Part model, mm, in its own coordinate system. A direction names the side the tool comes from. Give positions to 0.01 mm unless a question says otherwise; leave off trailing zeros. Loops run counter-clockwise (first coordinate to the right, second up) from the corner with the lowest first, then second, coordinate; pieces in that order, holes last. Notation, with made-up numbers: M -15.75,50.25 L 35.25,50.25 A17 ccw 35.25,72.25 Z; hole C 62,-5.5 d10. An arc over 180 degrees is marked long. Answer in a Markdown table with one row per item.
from build123d import *

# Parameters (mm, degrees)
SKETCH_W     = 12.8
SKETCH_H     = 9.8
PAD_DEPTH    = 10
SKETCH001_W  = 15
SKETCH001_H  = 12
PAD001_DEPTH = 1
CHAMFER_SIZE = 1


with BuildPart() as part:
    # Sketch → Pad (new body)
    with BuildSketch(Plane.XZ):
        Rectangle(SKETCH_W, SKETCH_H)
    extrude(amount=PAD_DEPTH)

    # Sketch001 (on Face1 of Pad) → Pad001 (join)
    with BuildSketch(Plane(origin=(0, 0, 4.9), x_dir=(-1, 0, 0), z_dir=(0, 0, 1))):
        with Locations((-0.066966, 5)):
            Rectangle(SKETCH001_W, SKETCH001_H)
    extrude(amount=PAD001_DEPTH)

    # Chamfer
    chamfer_edges = [part.edges().sort_by_distance(p)[0] for p in [
        (-6.4, -10, 0),
        (0, -10, -4.9),
        (-6.4, -5, -4.9),
        (-6.4, 0, 0),
        (6.4, -10, 0),
        (6.4, -5, -4.9),
        (6.4, 0, 0),
        (0, 0, -4.9),
    ]]
    chamfer(chamfer_edges, length=CHAMFER_SIZE)


solid = part.part
(1) Pin check, flat tips, straight feed: pin 1 Ø4.5 at (x, z) = (2.5, 0.5) entering from -Y; pin 2 Ø2.5 at (y, z) = (-6, 2.5) entering from -X; pin 3 Ø2 at (x, z) = (0.5, 3.5) entering from +Y. Stop position of each tip, or through.
Recorded:
| item | result |
|---|---|
| pin 1 | stops at y = -10 |
| pin 2 | stops at x = -6.4 |
| pin 3 | stops at y = 0 |
(2) Saw through at C-C (x = -1.5). Write the cut outline in (y, z).
Recorded:
| item | result |
|---|---|
| outline | M -11,4.9 L -10,4.9 L -10,-3.9 L -9,-4.9 L -1,-4.9 L 0,-3.9 L 0,4.9 L 1,4.9 L 1,5.9 L -11,5.9 Z |
(3) Drill centre lines: line 1 along Y through (x, z) = (2.25, 4.5); line 2 along X through (y, z) = (-8.5, 3.5); line 3 along Z through (x, y) = (-6.5, -10). Where is each one in solid material? Low to high.
Recorded:
| item | result |
|---|---|
| line 1 | y = -10 to 0 |
| line 2 | x = -6.4 to 6.4 |
| line 3 | z = 4.9 to 5.9 |
(4) Which spindle directions (+Z, -Z, +X, -X, +Y, -Y) get a long thin tool onto all of the face, cutting with end or side? Do faces 1 (the face through (5.9, -0.5, 0.4)), 2 (the face through (6.4, -5, 0)), 3 (the face through (5.9, -9.5, 0.4)). Say none if no direction does.
Recorded:
| item | result |
|---|---|
| face 1 | -Z, +X, +Y |
| face 2 | -Z, +X, +Y, -Y |
| face 3 | -Z, +X, -Y |
(5) Saw through at B-B (z = -0.25). Write the cut outline in (x, y), plus the area to 3 significant figures.
Recorded:
| item | result |
|---|---|
| outline | M -6.4,-9 L -5.4,-10 L 5.4,-10 L 6.4,-9 L 6.4,-1 L 5.4,0 L -5.4,0 L -6.4,-1 Z |
| area | 126 mm^2 |
(6) Saw through at A-A (y = -3.5). Write the cut outline in (x, z), plus the area to 3 significant figures.
Recorded:
| item | result |
|---|---|
| outline | M -7.43,4.9 L -6.4,4.9 L -6.4,-3.9 L -5.4,-4.9 L 5.4,-4.9 L 6.4,-3.9 L 6.4,4.9 L 7.57,4.9 L 7.57,5.9 L -7.43,5.9 Z |
| area | 139 mm^2 |
